from build123d import *

# Parameters (mm, degrees)
SKETCH2_W           = 85
SKETCH2_H           = 5
BOSS_EXTRUDE1_DEPTH = 5
BOSS_EXTRUDE2_DEPTH = 5
LPATTERN1_COUNT     = 16
LPATTERN1_PITCH     = 3.142
SKETCH3_W           = 2
SKETCH3_H           = 4
BOSS_EXTRUDE3_DEPTH = 10


with BuildPart() as part:
    # Sketch2 → Boss-Extrude1 (new body)
    with BuildSketch(Plane(origin=(0, 0, 0), x_dir=(1, 0, 0), z_dir=(0, 1, 0))):
        with Locations((9.747191011, 2.5)):
            Rectangle(SKETCH2_W, SKETCH2_H)
    extrude(amount=BOSS_EXTRUDE1_DEPTH)

    # Sketch2_3 → Boss-Extrude2 (add)
    with BuildSketch(Plane(origin=(0, 0, 0), x_dir=(1, 0, 0), z_dir=(0, 1, 0))):
        with BuildLine():
            ThreePointArc((-26.933875962, 7.25), (-27.510500845, 6.185840671), (-27.752808989, 5))
            Line((-27.752808989, 5), (-25.752808989, 5))
            ThreePointArc((-25.752808989, 5), (-25.995117132, 6.185840671), (-26.571742016, 7.25))
            Line((-26.571742016, 7.25), (-26.933875962, 7.25))
        make_face()
    boss_extrude2 = extrude(amount=BOSS_EXTRUDE2_DEPTH)

    # LPattern1: Boss-Extrude2 ×16
    with Locations(*[(i * LPATTERN1_PITCH, 0, 0) for i in range(1, LPATTERN1_COUNT)]):
        add(boss_extrude2)

    # Sketch3 → Boss-Extrude3 (add)
    with BuildSketch(Plane.ZY.offset(32.752808989)):
        with Locations((-1.5, 2.5)):
            Rectangle(SKETCH3_W, SKETCH3_H)
    extrude(amount=BOSS_EXTRUDE3_DEPTH)


solid = part.part
Model file for the job. Use its own axes, mm. A direction names the side the tool comes from. Round coordinates to 2 decimals unless told otherwise and drop trailing zeros. Order: outer loops, then holes, each group sorted by start corner. A loop starts at its lowest first (then second) coordinate and runs counter-clockwise, first axis right, second up.
(1) Drill centre lines: line 1 (Z direction, x = 41.5, y = 3.3); line 2 (X direction, y = 2.8, z = -4); line 3 (Z direction, x = -36, y = 1.55). Where is each one in solid material? Low to high.
(2) Pin check, flat tips, straight feed: pin 1 (1.5 mm diameter, centred on x = 31, y = 2.5, fed in from -Z); pin 2 (1.6 mm diameter, centred on x = -39.5, z = -2, fed in from +Y); pin 3 (1.6 mm diameter, centred on x = -35.5, z = -1, fed in from -Y). Stop position of each tip, or through.
(3) Band-saw the part on B-B (x = 40.5). List the corners of the cut face in (y, z), then the cut area to 3 significant figures.
(4) Band-saw the part on A-A (z = -3.5). List the corners of the cut face in (x, y).
(5) 3-axis set-ups, long thin cutter, end or side, ignore diameter. For faces 1 (the face through (18, 2.46, -6.17)), 2 (the face through (9, 0, -3)): which of +Z, -Z, +X, -X, +Y, -Y reach the whole face in a straight line?
(6) Pull direction X, two halves, no side cores. Call faces 3 (the face through (-38, 4.5, -2)), 4 (the face through (-24.363, 2.465, -6.202)), 5 (the face through (52.247, 2, -2)): released by +X, released by -X, zero draft, split by the parting line, or undercut.
Verdict:
1. line 1: z = -5 to 0
1. line 2: x = -32.75 to 52.25
1. line 3: z = -2.5 to -0.5
2. pin 1: stops at z = -5
2. pin 2: stops at y = 4.5
2. pin 3: stops at y = 0.5
3. outline: (0, -5) - (5, -5) - (5, 0) - (0, 0) - close
3. area: 25.0 mm2
4. outline: (-32.75, 0) - (52.25, 0) - (52.25, 5) - (-32.75, 5) - close
5. face 1: -Z, +Y, -Y
5. face 2: +Z, -Z, +X, -X, -Y
6. face 3: zero draft
6. face 4: undercut
6. face 5: released by +X
